Check sheet for the drawn part. Datum: minimum x, y, z corner. Units: mm. A direction names the side the tool comes from. Round coordinates to 2 decimals unless told otherwise and drop trailing zeros. Write each loop counter-clockwise with the first axis right and the second up, starting at its lowest first coordinate (ties: lowest second). Pieces come first, ordered by that corner, then holes. Notation, with made-up numbers: (76.25, -17) - (132.25, -17) arc R20 ccw to (132.25, -10) - close; hole circle Ø3 at (20.5, -22). An arc over 180 degrees is marked (long way). Write each question's results on one line, items separated by ' | '.
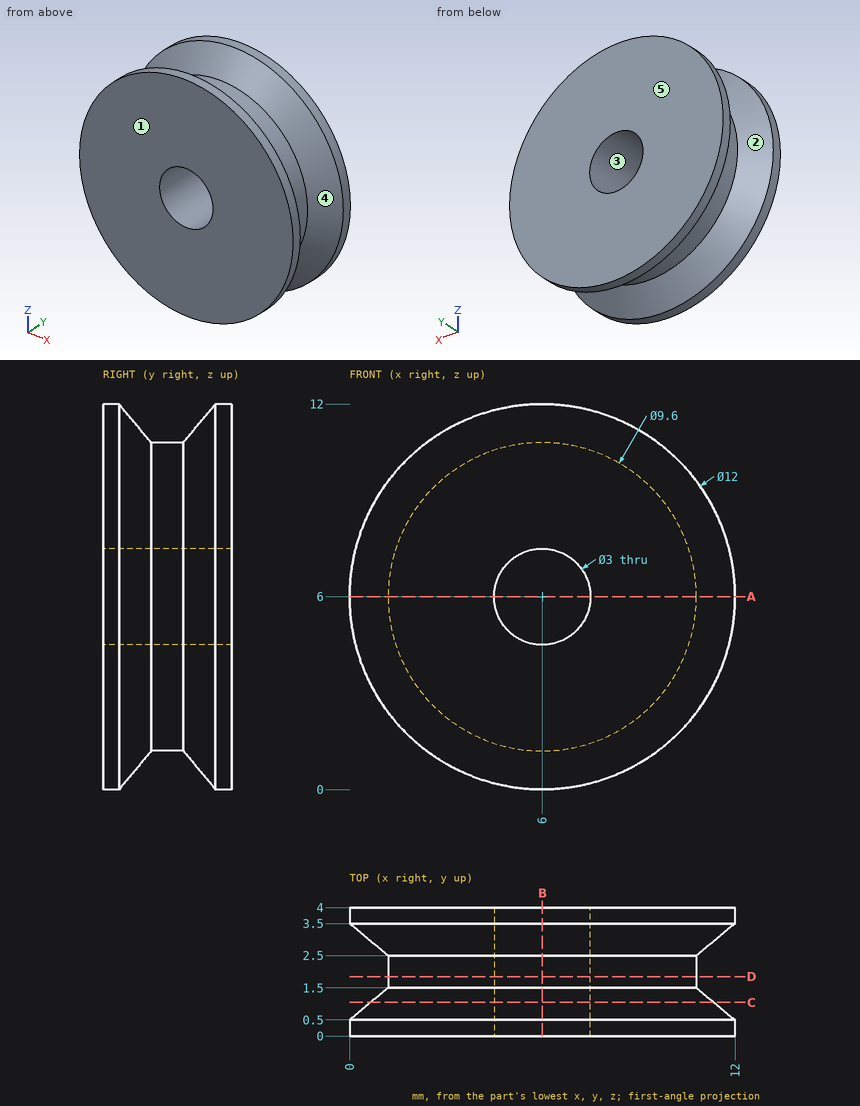
(1) Go/stop test with flat-tipped pins: pin 1 Ø1 at (x, y) = (4.5, 1.5) entering from -Z; pin 2 Ø1 at (y, z) = (1.5, 9.5) entering from -X. Record where each tip stops, or that it passes through.
Answer:
pin 1: z = 0.8 | pin 2: x = 1.79
(2) Thickness scan on L1, parallel to Z at x = 6, y = 2; L2, parallel to Z at x = 6, y = 2.55; L3, parallel to X at y = 1.3, z = 6. Record the ranges inside material, lowest first.
Answer:
L1: 1.2 to 4.5, 7.5 to 10.8 | L2: 1.14 to 4.5, 7.5 to 10.86 | L3: 0.96 to 4.5, 7.5 to 11.04
(3) Section check C-C (y = 1.05). Record the cut outline in (x, z), plus the area to 3 significant figures.
Answer:
outline: circle Ø10.68 at (6, 6); hole circle Ø3 at (6, 6) | area: 82.5 mm2
(4) Section check B-B (x = 6). Record the cut outline in (y, z), plus the area to 3 significant figures.
Answer:
outline: (0, 0) - (0.5, 0) - (1.5, 1.2) - (2.5, 1.2) - (3.5, 0) - (4, 0) - (4, 4.5) - (0, 4.5) - close; (0, 7.5) - (4, 7.5) - (4, 12) - (3.5, 12) - (2.5, 10.8) - (1.5, 10.8) - (0.5, 12) - (0, 12) - close | area: 31.2 mm2
(5) Section check A-A (z = 6). Record the cut outline in (x, y), plus the area to 3 significant figures.
Answer:
outline: (0, 0) - (4.5, 0) - (4.5, 4) - (0, 4) - (0, 3.5) - (1.2, 2.5) - (1.2, 1.5) - (0, 0.5) - close; (7.5, 0) - (12, 0) - (12, 0.5) - (10.8, 1.5) - (10.8, 2.5) - (12, 3.5) - (12, 4) - (7.5, 4) - close | area: 31.2 mm2
(6) Mould release check, pull along Y, two halves, no side actions. Record for the marked faces 1, 2 and 3: released by +Y, released by -Y, zero draft, split by the parting line, or undercut.
Answer:
face 1: released by -Y | face 2: undercut | face 3: zero draft
(7) Set-up check for the marked faces 4 and 5: record each of +Z, -Z, +X, -X, +Y, -Y from which the full face is reachable in a straight line by a thin tool's end or side.
Answer:
face 4: none | face 5: +Z, -Z, +X, -X, +Y
(8) Section check D-D (y = 1.85). Record the cut outline in (x, z), plus the area to 3 significant figures.
Answer:
outline: circle Ø9.6 at (6, 6); hole circle Ø3 at (6, 6) | area: 65.3 mm2
